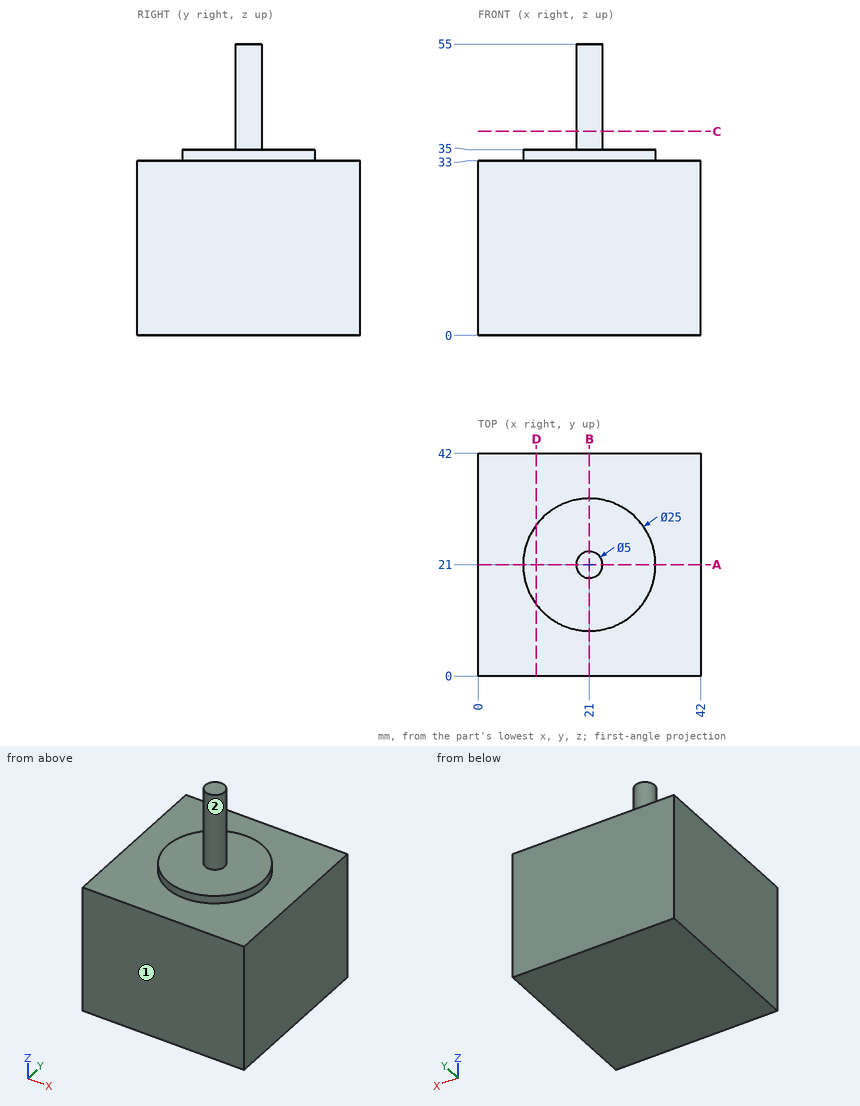
Here's the drawing with two shaded views (mm, measured from the low corner). I have some questions. A direction names the side the tool comes from. Round coordinates to 2 decimals unless told otherwise and drop trailing zeros. Write each loop counter-clockwise with the first axis right and the second up, starting at its lowest first coordinate (ties: lowest second). Pieces come first, ordered by that corner, then holes. Notation, with made-up numbers: M 43,47 L 55,47 A33 ccw 55,84 Z; hole C -35,-27 d1. An arc over 180 degrees is marked long. Answer in a Markdown table with one row per item. Add a question column.
Q1. Will this pin go through, and if not, where does the flat tip stop? pin 1 Ø12 at (x, y) = (29, 14.5) entering from +Z.
Q2. On a 3-axis mill with a long thin cutter (end or side, diameter ignored), from which of +Z, -Z, +X, -X, +Y, -Y can I reach the whole of each face in a straight line? I mean the marked faces 1 and 2. Say none if no direction works.
Q3. Imagine slicing it at C-C (z = 38.5). Please give me the cut outline in (x, y).
Q4. Imagine slicing it at A-A (y = 21). Please give me the cut outline in (x, z), then the cut area to 3 significant figures.
Q5. If I drill on line 1 (Z direction, x = 10, y = 26.5); line 2 (Z direction, x = 40.5, y = 3); line 3 (X direction, y = 27.5, z = 34), over which ranges is the centre line in solid material (lowest first)? Write a range as from..to.
Q6. Imagine slicing it at D-D (x = 11). Please give me the cut outline in (y, z), then the cut area to 3 significant figures.
Values:
| question | item | result |
|---|---|---|
| 1 | pin 1 | z = 35 |
| 2 | face 1 | +Z, -Z, +X, -X, -Y |
| 2 | face 2 | +Z |
| 3 | outline | C 21,21 d5 |
| 4 | outline | M 0,0 L 42,0 L 42,33 L 33.5,33 L 33.5,35 L 23.5,35 L 23.5,55 L 18.5,55 L 18.5,35 L 8.5,35 L 8.5,33 L 0,33 Z |
| 4 | area | 1,540 mm^2 |
| 5 | line 1 | 0..35 |
| 5 | line 2 | 0..33 |
| 5 | line 3 | 10.32..31.68 |
| 6 | outline | M 0,0 L 42,0 L 42,33 L 28.5,33 L 28.5,35 L 13.5,35 L 13.5,33 L 0,33 Z |
| 6 | area | 1,420 mm^2 |
